Answer from the drawing. Dimensions are ordinates in mm from the lowest x, y and z of the part. Coordinates: 2 decimals unless noted, no trailing zeros. Order: outer loops, then holes, each group sorted by start corner. A loop starts at its lowest first (then second) coordinate and runs counter-clockwise, first axis right, second up. Notation, with made-up numbers: (57, 66.5) -> (93, 66.5) arc R22 ccw to (93, 105.5) -> close; hole circle Ø7 at (5, 40). An arc over 180 degrees is marked (long way). Answer in a Markdown table with one row per item.
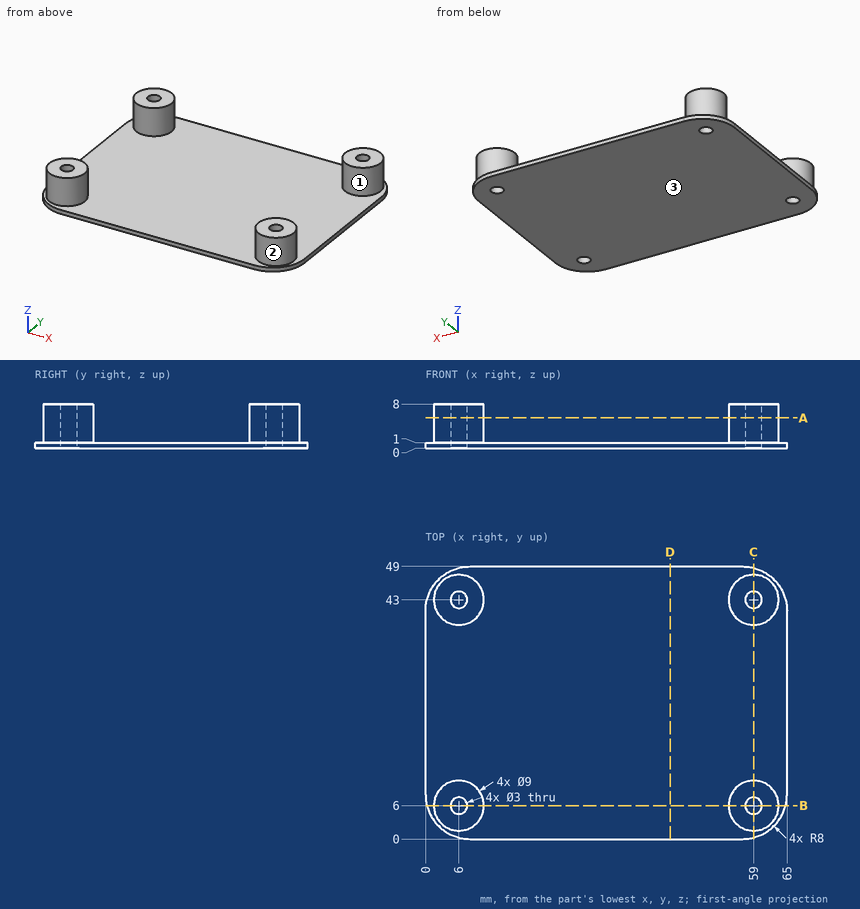
Q1. Consider line 1 (Y direction, x = 6, z = 5); line 2 (Y direction, x = 58, z = 4); line 3 (Z direction, x = 61, y = 38). Determine where each line is inside the solid, lowest interval first.
Outcome:
| item | result |
|---|---|
| line 1 | 1.5 to 4.5, 7.5 to 10.5, 38.5 to 41.5, 44.5 to 47.5 |
| line 2 | 1.61 to 4.88, 7.12 to 10.39, 38.61 to 41.88, 44.12 to 47.39 |
| line 3 | 0 to 1 |
Q2. The part is cut by section A-A (z = 5.5). Write down the section's boundary in (x, y).
Outcome:
| item | result |
|---|---|
| outline | circle Ø9 at (6, 6); circle Ø9 at (6, 43); circle Ø9 at (59, 6); circle Ø9 at (59, 43); hole circle Ø3 at (6, 6); hole circle Ø3 at (6, 43); hole circle Ø3 at (59, 6); hole circle Ø3 at (59, 43) |
Q3. Given pin 1 (14.5 mm diameter, centred on x = 31.5, y = 27.5, fed in from +Z); pin 2 (3.5 mm diameter, centred on x = 59, y = 6, fed in from -Z); pin 3 (4 mm diameter, centred on y = 10.5, z = 7, fed in from -X); pin 4 (4 mm diameter, centred on y = 5.5, z = 2.5, fed in from +X), each flat-ended and moving along its own axis, determine where each tip first touches the part or whether it passes through.
Outcome:
| item | result |
|---|---|
| pin 1 | z = 1 |
| pin 2 | z = 0 |
| pin 3 | x = 2.26 |
| pin 4 | x = 64.91 |
Q4. For a pull along X with two mould halves and no side action, classify the marked faces 1, 2 and 3 as pulls with the +X half, pulls with the -X half, needs draft (parallel to the pull), parting line crosses it, or undercut.
Outcome:
| item | result |
|---|---|
| face 1 | undercut |
| face 2 | undercut |
| face 3 | needs draft |
Q5. The part is cut by section C-C (x = 59). Write down the section's boundary in (y, z), then the cut area to 3 significant figures.
Outcome:
| item | result |
|---|---|
| outline | (0.25, 0) -> (4.5, 0) -> (4.5, 8) -> (1.5, 8) -> (1.5, 1) -> (0.25, 1) -> close; (7.5, 0) -> (41.5, 0) -> (41.5, 8) -> (38.5, 8) -> (38.5, 1) -> (10.5, 1) -> (10.5, 8) -> (7.5, 8) -> close; (44.5, 0) -> (48.75, 0) -> (48.75, 1) -> (47.5, 1) -> (47.5, 8) -> (44.5, 8) -> close |
| area | 126 mm² |
Q6. The part is cut by section B-B (y = 6). Write down the section's boundary in (x, z), then the cut area to 3 significant figures.
Outcome:
| item | result |
|---|---|
| outline | (0.25, 0) -> (4.5, 0) -> (4.5, 8) -> (1.5, 8) -> (1.5, 1) -> (0.25, 1) -> close; (7.5, 0) -> (57.5, 0) -> (57.5, 8) -> (54.5, 8) -> (54.5, 1) -> (10.5, 1) -> (10.5, 8) -> (7.5, 8) -> close; (60.5, 0) -> (64.75, 0) -> (64.75, 1) -> (63.5, 1) -> (63.5, 8) -> (60.5, 8) -> close |
| area | 142 mm² |
Q7. The part is cut by section D-D (x = 44). Write down the section's boundary in (y, z).
Outcome:
| item | result |
|---|---|
| outline | (0, 0) -> (49, 0) -> (49, 1) -> (0, 1) -> close |
